Could you check a few things on this model? Use its own coordinates, in mm. A direction names the side the tool comes from. Coordinates: 2 decimals unless noted, no trailing zeros. Order: outer loops, then holes, each group sorted by start corner. A loop starts at its lowest first (then second) coordinate and runs counter-clockwise, first axis right, second up. Notation, with made-up numbers: (-2, 42.25) - (55, 42.25) arc R32 ccw to (55, 76.25) - close; hole circle Ø7 at (-28.75, 22). An arc over 180 degrees is marked (long way). Answer as a JSON object with one key per item and string values. Group by question number.
(1) Which directions (+Z, -Z, +X, -X, +Y, -Y) give clear straight access to the entire face, cutting with the end or side of a thin tool? Please do faces 1 (the flat face through (52, 15, -10)), 2 (the cylindrical face through (-297.15, 14.08, -56.99)), 3 (the flat face through (-250, 10, 1)).
(2) Will these pins go through, and if not, where does the flat tip stop? P1, Ø9, axis at x = 56.5, z = -23.5, coming from the +Y side; P2, Ø11, axis at y = 16.5, z = 23, coming from the -X side.
(3) We'd pull the mould along X, two halves only. Please class faces 4 (the flat face through (-275, 5, -55)), 5 (the flat face through (280, 15, 25)), 6 (the flat face through (-275, 12, 50)): pulls with the +X half, pulls with the -X half, needs draft (parallel to the pull), parting line crosses it, or undercut.
(4) Please list where these lines run through material, in increasing order: probe 1 along Z at (x, y) = (-45, 15.5); probe 2 along X at (y, z) = (14.5, -15); probe 3 along Y at (x, z) = (94.5, -34.5).
(5) Imagine slicing it at B-B, the plane y = 13.75. Write out the boundary of the cut face in (x, z).
(6) Imagine slicing it at A-A, the plane z = -29.5. Write out the boundary of the cut face in (x, y).
(7) Imagine slicing it at D-D, the plane z = 3. Write out the boundary of the cut face in (x, y).
(8) Imagine slicing it at C-C, the plane x = -14.5. Write out the boundary of the cut face in (y, z), and give its area (3 significant figures).
from build123d import *

# Parameters (mm, degrees)
SKETCH1_W           = 600
SKETCH1_H           = 120
BOSS_EXTRUDE1_DEPTH = 20
CUT_EXTRUDE1_REACH  = 325.728
SKETCH6_W           = 450
SKETCH6_H           = 30
CUT_EXTRUDE2_DEPTH  = 10
FILLET1_R           = 10
FILLET2_R           = 5
CUT_EXTRUDE3_REACH  = 308.594
SKETCH7_W           = 50
SKETCH7_H           = 100


with BuildPart() as part:
    # Sketch1 → Boss-Extrude1 (new body)
    with BuildSketch(Plane(origin=(0, 0, 0), x_dir=(1, 0, 0), z_dir=(0, 1, 0))):
        Rectangle(SKETCH1_W, SKETCH1_H)
    extrude(amount=BOSS_EXTRUDE1_DEPTH)

    # Sketch4 → Cut-Extrude1 (cut, up to next)
    with BuildSketch(Plane.XY.offset(60), mode=Mode.PRIVATE) as cut_extrude1_sk1:
        Polygon((-300, 10), (-250, 0), (-300, 0), align=None)
    cut_extrude1_tool1 = extrude(cut_extrude1_sk1.sketch, amount=-CUT_EXTRUDE1_REACH, mode=Mode.PRIVATE) & part.part
    add(cut_extrude1_tool1.solids().sort_by_distance((-283.333333, 3.333333, 60))[0], mode=Mode.SUBTRACT)

    # Sketch6 → Cut-Extrude2 (cut)
    with BuildSketch(Plane(origin=(0, 20, 0), x_dir=(1, 0, 0), z_dir=(0, 1, 0))):
        with Locations((55, 25)):
            Rectangle(SKETCH6_W, SKETCH6_H)
        with Locations((55, -25)):
            Rectangle(SKETCH6_W, SKETCH6_H)
    extrude(amount=-CUT_EXTRUDE2_DEPTH, mode=Mode.SUBTRACT)

    # Fillet1
    fillet1_edges = [part.edges().sort_by_distance(p)[0] for p in [
        (-300, 15, -60),
        (300, 10, -60),
        (300, 10, 60),
        (-300, 15, 60),
    ]]
    fillet(fillet1_edges, radius=FILLET1_R)

    # Fillet2
    fillet2_edges = [part.edges().sort_by_distance(p)[0] for p in [
        (-170, 15, -10),
        (-170, 15, -40),
        (280, 15, -40),
        (280, 15, -10),
        (-170, 15, 40),
        (-170, 15, 10),
        (280, 15, 10),
        (280, 15, 40),
    ]]
    fillet(fillet2_edges, radius=FILLET2_R)

    # Sketch7 → Cut-Extrude3 (cut, up to next)
    with BuildSketch(Plane(origin=(0, 20, 0), x_dir=(1, 0, 0), z_dir=(0, 1, 0)), mode=Mode.PRIVATE) as cut_extrude3_sk1:
        with Locations((-275, 0)):
            Rectangle(SKETCH7_W, SKETCH7_H)
    cut_extrude3_tool1 = extrude(cut_extrude3_sk1.sketch, amount=-CUT_EXTRUDE3_REACH, mode=Mode.PRIVATE) & part.part
    add(cut_extrude3_tool1.solids().sort_by_distance((-275, 20, 0))[0], mode=Mode.SUBTRACT)


solid = part.part
Result set:
{
 "1": {"face 1": "+Y", "face 2": "-Z, -X, +Y, -Y", "face 3": "-X, +Y, -Y"},
 "2": {"P1": "stops at y = 10", "P2": "stops at x = -250"},
 "3": {"face 4": "pulls with the -X half", "face 5": "undercut", "face 6": "needs draft"},
 "4": {"probe 1": "z = -60 to -40, -10 to 10, 40 to 60", "probe 2": "x = -250 to -170, 280 to 300", "probe 3": "y = 0 to 10"},
 "5": {"outline": "(-300, -50) arc R10 ccw to (-290, -60) - (290, -60) arc R10 ccw to (300, -50) - (300, 50) arc R10 ccw to (290, 60) - (-290, 60) arc R10 ccw to (-300, 50) - (-250, 50) - (-250, -50) - close; hole (-170, -35) arc R5 ccw to (-165, -40) - (275, -40) arc R5 ccw to (280, -35) - (280, -15) arc R5 ccw to (275, -10) - (-165, -10) arc R5 ccw to (-170, -15) - close; hole (-170, 15) arc R5 ccw to (-165, 10) - (275, 10) arc R5 ccw to (280, 15) - (280, 35) arc R5 ccw to (275, 40) - (-165, 40) arc R5 ccw to (-170, 35) - close"},
 "6": {"outline": "(-250, 0) - (300, 0) - (300, 20) - (280, 20) - (280, 10) - (-170, 10) - (-170, 20) - (-250, 20) - close"},
 "7": {"outline": "(-250, 0) - (300, 0) - (300, 20) - (-250, 20) - close"},
 "8": {"outline": "(0, -60) - (20, -60) - (20, -40) - (10, -40) - (10, -10) - (20, -10) - (20, 10) - (10, 10) - (10, 40) - (20, 40) - (20, 60) - (0, 60) - close", "area": "1,800 mm^2"}
}
